Here's how the part is built. I have some questions about the finished solid (model axes, mm). Coordinates: 2 decimals unless noted, no trailing zeros. Write each loop counter-clockwise with the first axis right and the second up, starting at its lowest first coordinate (ties: lowest second). Pieces come first, ordered by that corner, then holes.
Item 1: If I drill on line 1 (Z direction, x = 160, y = 1.9); line 2 (X direction, y = 2, z = 91.5), over which ranges is the centre line in solid material (lowest first)?
Item 2: I'm going to push a flat-ended pin straight in: pin 1 Ø2 at (x, y) = (198, 4.5) entering from -Z. Where does the tip first touch, or does it pass through?
Item 3: If we section it at A-A (x = 136): Please give me the cut outline in (y, z), then the cut area to 3 significant figures.
Item 4: If we section it at B-B (y = 4.55): Please give me the cut outline in (x, z), then the cut area to 3 significant figures.
Item 5: If we section it at C-C (z = 98): Please give me the cut outline in (x, y), then the cut area to 3 significant figures.
Autodesk Fusion 360 part; units mm, degrees
sketch "Unsorted Smarties Back" plane through (0, 0, 0) normal (0, 1, 0) x (1, 0, 0)
  line L0 (0, 0) -> (270, 0)
  line L1 (270, 0) -> (270, -161)
  line L2 (270, -161) -> (0, -161)
  line L3 (0, -161) -> (0, 0)
  dimension "d1" = 270
  dimension "d2" = 161
extrude "Extrude1" add sketch "Unsorted Smarties Back" along normal blind 6
sketch "Smartie Feed" plane through (0, 0, 0) normal (0, -1, 0) x (1, 0, 0)
  line L0 (270, 161) -> (0, 161)
  line L1 (0, 161) -> (0, 0)
  line L2 (0, 0) -> (270, 0)
  line L3 (270, 0) -> (270, 161)
  line L4 (90, 120) -> (180, 120)
  line L5 (180, 120) -> (180, 90)
  line L6 (180, 90) -> (90, 90)
  line L7 (90, 90) -> (90, 120)
  dimension "d6" = 90
  dimension "d7" = 90
  dimension "d8" = 41
  dimension "d9" = 30
  dimension "d12" = 90
extrude "Extrude2" cut sketch "Smartie Feed" against normal blind 6 contours L4 L5 L6 L7
equation "mdfThickness = 6 mm"
equation "d4 = mdfThickness"
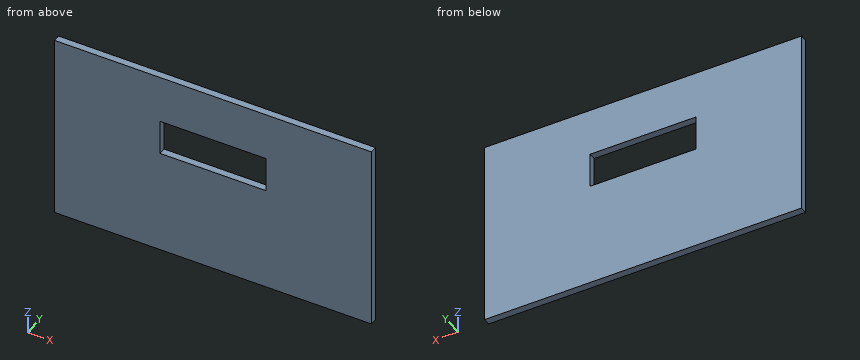
Answer list:
1. line 1: z = 0 to 90, 120 to 161
1. line 2: x = 0 to 90, 180 to 270
2. pin 1: stops at z = 0
3. outline: (0, 0) - (6, 0) - (6, 90) - (0, 90) - close; (0, 120) - (6, 120) - (6, 161) - (0, 161) - close
3. area: 786 mm2
4. outline: (0, 0) - (270, 0) - (270, 161) - (0, 161) - close; hole (90, 90) - (180, 90) - (180, 120) - (90, 120) - close
4. area: 40,800 mm2
5. outline: (0, 0) - (90, 0) - (90, 6) - (0, 6) - close; (180, 0) - (270, 0) - (270, 6) - (180, 6) - close
5. area: 1,080 mm2
